Geometry check sheet. Reference: the model listing, model coordinates, mm. A direction names the side the tool comes from. Round coordinates to 2 decimals unless told otherwise and drop trailing zeros. Write each loop counter-clockwise with the first axis right and the second up, starting at its lowest first coordinate (ties: lowest second). Pieces come first, ordered by that corner, then holes. Notation, with made-up numbers: M 89,65.5 L 136,65.5 A10 cw 136,76.5 Z; hole C 57,-22 d3. An arc over 180 degrees is marked long. Answer in a Markdown table with one row per item. Add a question column.
from build123d import *

# Parameters (mm, degrees)
ESQUISSE1_R        = 4.25
BOSS_EXTRU_1_DEPTH = 1.5
ESQUISSE1_2_R      = 5.75
ESQUISSE1_2_R_2    = 4.25
EXTRU_MINCE1_DEPTH = 80
ESQUISSE2_R        = 5.75
ESQUISSE2_R_2      = 4.25
BOSS_EXTRU_2_DEPTH = 3
ESQUISSE4_W        = 57
ESQUISSE4_H        = 83
ESQUISSE4_R        = 3.05
BOSS_EXTRU_3_DEPTH = 3
CONG_1_R           = 5


with BuildPart() as part:
    # Esquisse1 → Boss.-Extru.1 (new body)
    with BuildSketch(Plane.XY):
        Circle(ESQUISSE1_R)
    extrude(amount=BOSS_EXTRU_1_DEPTH)

    # Esquisse1<2> → Extru.-Mince1 (add)
    with BuildSketch(Plane.XY):
        Circle(ESQUISSE1_2_R)
        Circle(ESQUISSE1_2_R_2, mode=Mode.SUBTRACT)
    extrude(amount=EXTRU_MINCE1_DEPTH)

    # Esquisse2 → Boss.-Extru.2 (add)
    # profile 1 of 3: a face of its own
    with BuildSketch(Plane.XY.offset(80)):
        with BuildLine():
            Line((9.78589137, 2.851632123), (1.78589137, 5.465628236))
            ThreePointArc((1.78589137, 5.465628236), (4.654641521, 3.375916514), (5.75, 0))
            ThreePointArc((5.75, 0), (4.654641521, -3.375916514), (1.78589137, -5.465628236))
            Line((1.78589137, -5.465628236), (9.78589137, -2.851632123))
            ThreePointArc((9.78589137, -2.851632123), (11.282630579, -1.761347746), (11.85412196, 0))
            ThreePointArc((11.85412196, 0), (11.282630579, 1.761347746), (9.78589137, 2.851632123))
        make_face()
    # profile 2 of 3: a face of its own
    with BuildSketch(Plane.XY.offset(80)):
        with BuildLine():
            ThreePointArc((-1.78589137, -5.465628236), (-5.75, 0), (-1.78589137, 5.465628236))
            Line((-1.78589137, 5.465628236), (-9.78589137, 2.851632123))
            ThreePointArc((-9.78589137, 2.851632123), (-11.282630579, 1.761347746), (-11.85412196, 0))
            ThreePointArc((-11.85412196, 0), (-11.282630579, -1.761347746), (-9.78589137, -2.851632123))
            Line((-9.78589137, -2.851632123), (-1.78589137, -5.465628236))
        make_face()
    # profile 3 of 3: a face of its own
    with BuildSketch(Plane.XY.offset(80)):
        with Locations(Location((0, 0, 0), (0, 0, 108.094778376))):
            Circle(ESQUISSE2_R)
        Circle(ESQUISSE2_R_2, mode=Mode.SUBTRACT)
    extrude(amount=BOSS_EXTRU_2_DEPTH)

    # Esquisse4 → Boss.-Extru.3 (add)
    with BuildSketch(Plane(origin=(0, -4.5, 0), x_dir=(1, 0, 0), z_dir=(0, 1, 0))):
        with Locations((0, -41.5)):
            Rectangle(ESQUISSE4_W, ESQUISSE4_H)
        with Locations(Location((22, -55, 0), (0, 0, 270))):
            Circle(ESQUISSE4_R, mode=Mode.SUBTRACT)
        with Locations(Location((-22, -55, 0), (0, 0, 270))):
            Circle(ESQUISSE4_R, mode=Mode.SUBTRACT)
        with Locations(Location((-22, -10, 0), (0, 0, 270))):
            Circle(ESQUISSE4_R, mode=Mode.SUBTRACT)
        with Locations(Location((22, -10, 0), (0, 0, 270))):
            Circle(ESQUISSE4_R, mode=Mode.SUBTRACT)
    extrude(amount=-BOSS_EXTRU_3_DEPTH)

    # Congé1
    # the kernel refuses this fillet: 5 mm, written as the material it adds along each edge
    with BuildSketch(Plane(origin=(3.579455266, -4.5, 97.897276329), x_dir=(0.4133759504867887, 0.9105604447586902, 0), z_dir=(0, 0, -1))) as cong_1_piece_1_section:
        with BuildLine():
            CenterArc((7.512123669, 4.451741005), CONG_1_R, 155.582916087, 87.334118235)
            Line((2.959321445, 6.518620758), (0, 0))
            ThreePointArc((0, 0), (2.617861279, 0.630497844), (5.235722557, 0))
        make_face()
    cong_1_piece_1 = extrude(amount=97.897276329, mode=Mode.PRIVATE)
    cong_1_piece_1 = split(cong_1_piece_1, bisect_by=Plane(origin=(6.241297516, -3.427571976, 83), z_dir=(0, 0, -1)), keep=Keep.TOP, mode=Mode.PRIVATE)
    add(cong_1_piece_1)
    with BuildSketch(Plane(origin=(-3.579455266, -4.5, 97.897276329), x_dir=(-0.41337595048678866, 0.9105604447586904, 0), z_dir=(0, 0, -1))) as cong_1_piece_2_section:
        with BuildLine():
            CenterArc((7.512123669, -4.451741005), CONG_1_R, 117.082965678, 87.334118235)
            Line((2.959321445, -6.518620758), (0, 0))
            ThreePointArc((0, 0), (2.617861279, -0.630497844), (5.235722557, 0))
        make_face()
    cong_1_piece_2 = extrude(amount=97.897276329, mode=Mode.PRIVATE)
    cong_1_piece_2 = split(cong_1_piece_2, bisect_by=Plane(origin=(-6.241297516, -3.427571976, 83), z_dir=(0, 0, -1)), keep=Keep.TOP, mode=Mode.PRIVATE)
    add(cong_1_piece_2)


solid = part.part
Item 1: Mould release check, pull along Y, two halves, no side actions. Record for faces 1 (the cylindrical face through (22.134, -5.979, 6.953)), 2 (the flat face through (0, -7.5, 41)), 3 (the flat face through (8.758, -3.188, 81.479)): +Y half, -Y half, draft (parallel to the pull), parting line (faces both ways), or undercut.
Item 2: Scan lines: probe 1 along X at (y, z) = (-6.8, 10); probe 2 along Y at (x, z) = (0, 42); probe 3 along Y at (x, z) = (-24, 72). Record each from-to range of solid material in increasing order. Write a range as from..to.
Item 3: Section check A-A, the plane z = 10. Record the boundary of the cut face in (x, y), and give its area (3 significant figures).
Item 4: Section check C-C, the plane z = 67.5. Record the boundary of the cut face in (x, y).
Item 5: Access from +Z, -Z, +X, -X, +Y, -Y to the whole of each face (thin tool, end or side, straight path). Record for faces 4 (the flat face through (-1, -4, 0)), 5 (the flat face through (0, 0, 1.5)), 6 (the flat face through (8, 0, 80)), 7 (the flat face through (-8, 1, 80)).
Item 6: Section check D-D, the plane y = -2. Record the boundary of the cut face in (x, z).
Item 7: Section check B-B, the plane x = 22. Record the boundary of the cut face in (y, z).
Item 8: Gauge pin test, flat ends, axial feed: pin 1 Ø5.5 at (x, z) = (22, 55) entering from -Y; pin 2 Ø8 at (x, z) = (-19.5, 9.5) entering from +Y; pin 3 Ø1.5 at (y, z) = (-2.5, 9.5) entering from -X; pin 4 Ø19.5 at (x, z) = (-16.5, 55) entering from +Y. Record the tip position at first contact, or that the pin passes through.
Result sheet:
| question | item | result |
|---|---|---|
| 1 | face 1 | draft |
| 1 | face 2 | -Y half |
| 1 | face 3 | undercut |
| 2 | probe 1 | x = -28.5..-25.05, -18.95..18.95, 25.05..28.5 |
| 2 | probe 2 | y = -7.5..-4.25, 4.25..5.75 |
| 2 | probe 3 | y = -7.5..-4.5 |
| 3 | outline | M -28.5,-7.5 L -25.05,-7.5 L -25.05,-4.5 L -28.5,-4.5 Z; M -18.95,-7.5 L 18.95,-7.5 L 18.95,-4.5 L 10.74,-4.5 A5 cw 5.74,0.27 A5.75 ccw -5.74,0.27 A5 cw -10.74,-4.5 L -18.95,-4.5 Z; M 25.05,-7.5 L 28.5,-7.5 L 28.5,-4.5 L 25.05,-4.5 Z; hole C 0,0 d8.5 |
| 3 | area | 192 mm^2 |
| 4 | outline | M -28.5,-7.5 L 28.5,-7.5 L 28.5,-4.5 L 10.74,-4.5 A5 cw 5.74,0.27 A5.75 ccw -5.74,0.27 A5 cw -10.74,-4.5 L -28.5,-4.5 Z; hole C 0,0 d8.5 |
| 5 | face 4 | -Z, +X, -X, +Y, -Y |
| 5 | face 5 | +Z |
| 5 | face 6 | -Z, +X, +Y |
| 5 | face 7 | -Z, -X, +Y |
| 6 | outline | M -11.09,80 L -6.41,80 L -6.41,0 L 6.41,0 L 6.41,80 L 11.09,80 L 11.09,83 L 3.75,83 L 3.75,1.5 L -3.75,1.5 L -3.75,83 L -11.09,83 Z |
| 7 | outline | M -7.5,0 L -4.5,0 L -4.5,6.95 L -7.5,6.95 Z; M -7.5,13.05 L -4.5,13.05 L -4.5,51.95 L -7.5,51.95 Z; M -7.5,58.05 L -4.5,58.05 L -4.5,83 L -7.5,83 Z |
| 8 | pin 1 | passes through |
| 8 | pin 2 | stops at y = -4.5 |
| 8 | pin 3 | stops at x = -7.43 |
| 8 | pin 4 | stops at y = -2.52 |
